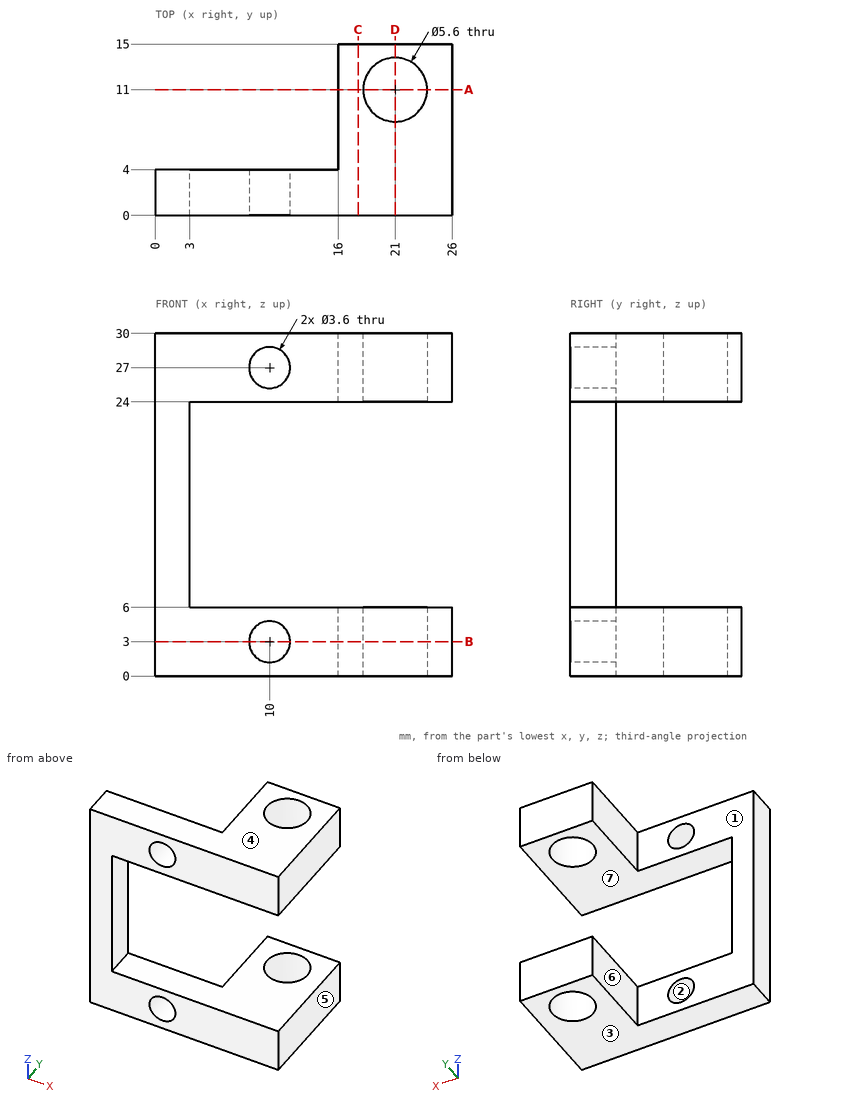
Drawing for the job (mm, zero at the part's lowest x, y, z). A direction names the side the tool comes from. Give positions to 0.01 mm unless a question says otherwise; leave off trailing zeros. Write each loop counter-clockwise with the first axis right and the second up, starting at its lowest first coordinate (ties: lowest second). Pieces come first, ordered by that corner, then holes. Notation, with made-up numbers: M -19.75,57 L 0.25,57 A11 ccw 0.25,78 Z; hole C 85,56 d4. An arc over 180 degrees is marked long. Return JSON: item names as keys, results as strings. Group by question number.
(1) Band-saw the part on B-B (z = 3). Give the cut face in (x, y), and give its area (3 significant figures).
(2) Mould opens along Z. For the marked faces 1, 2, 3 and 4 say: pulls with the +Z half, pulls with the -Z half, needs draft (parallel to the pull), parting line crosses it, or undercut.
(3) Band-saw the part on A-A (y = 11). Give the cut face in (x, z), and give its area (3 significant figures).
(4) Flat gauge pins, fed straight in: pin 1 Ø1.8 at (y, z) = (9, 1.5) entering from -X; pin 2 Ø13 at (x, z) = (7.5, 16.5) entering from +Y; pin 3 Ø3 at (y, z) = (2.5, 13) entering from +X. Where does each tip first touch, or does it go through?
(5) Band-saw the part on D-D (x = 21). Give the cut face in (y, z).
(6) Drill centre lines: L1, parallel to Z at x = 10, y = 1.6; L2, parallel to Y at x = 21, z = 4.15; L3, parallel to Z at x = 18, y = 11.5. Where is each one in solid material? Low to high. Write a range as [from, to].
(7) 3-axis set-ups, long thin cutter, end or side, ignore diameter. For the marked faces 5, 6 and 7: which of +Z, -Z, +X, -X, +Y, -Y reach the whole face in a straight line?
(8) Band-saw the part on C-C (x = 17.75). Give the cut face in (y, z), and give its area (3 significant figures).
Entries:
{
 "1": {"outline": "M 0,0 L 8.2,0 L 8.2,4 L 0,4 Z; M 11.8,0 L 26,0 L 26,15 L 16,15 L 16,4 L 11.8,4 Z; hole C 21,11 d5.6", "area": "175 mm^2"},
 "2": {"face 1": "needs draft", "face 2": "undercut", "face 3": "pulls with the -Z half", "face 4": "pulls with the +Z half"},
 "3": {"outline": "M 16,0 L 18.2,0 L 18.2,6 L 16,6 Z; M 16,24 L 18.2,24 L 18.2,30 L 16,30 Z; M 23.8,0 L 26,0 L 26,6 L 23.8,6 Z; M 23.8,24 L 26,24 L 26,30 L 23.8,30 Z", "area": "52.8 mm^2"},
 "4": {"pin 1": "stops at x = 16", "pin 2": "stops at y = 4", "pin 3": "stops at x = 3"},
 "5": {"outline": "M 0,0 L 8.2,0 L 8.2,6 L 0,6 Z; M 0,24 L 8.2,24 L 8.2,30 L 0,30 Z; M 13.8,0 L 15,0 L 15,6 L 13.8,6 Z; M 13.8,24 L 15,24 L 15,30 L 13.8,30 Z"},
 "6": {"L1": "z = [0, 1.2], [4.8, 6], [24, 25.2], [28.8, 30]", "L2": "y = [0, 8.2], [13.8, 15]", "L3": "z = [0, 6], [24, 30]"},
 "7": {"face 5": "+Z, -Z, +X, +Y, -Y", "face 6": "+Z, -Z, -X, +Y", "face 7": "+X, +Y, -Y"},
 "8": {"outline": "M 0,0 L 15,0 L 15,6 L 0,6 Z; M 0,24 L 15,24 L 15,30 L 0,30 Z", "area": "180 mm^2"}
}
